```python
from build123d import *

# Parameters (mm, degrees)
CROQUIS1_R              = 9
SALIENTE_EXTRUIR1_DEPTH = 8
CROQUIS3_R              = 11
SALIENTE_EXTRUIR2_DEPTH = 1
SALIENTE_EXTRUIR3_START = 1
CROQUIS4_R              = 11
SALIENTE_EXTRUIR3_DEPTH = 1
CROQUIS5_R              = 4.5
SALIENTE_EXTRUIR4_DEPTH = 6
CROQUIS6_R              = 2.5
CORTAR_EXTRUIR1_DEPTH   = 23.315913604
CROQUIS7_R              = 1
CORTAR_EXTRUIR2_DEPTH   = 18.972200756
CROQUIS8_R              = 1
CORTAR_EXTRUIR5_DEPTH   = 8
MATRIZC1_COUNT          = 20
CHAFL_N1_SIZE           = 0.5


with BuildPart() as part:
    # Croquis1 → Saliente-Extruir1 (new body)
    with BuildSketch(Plane(origin=(0, 0, 0), x_dir=(1, 0, 0), z_dir=(0, 1, 0))):
        with Locations(Location((0, 0, 0), (0, 0, 270))):
            Circle(CROQUIS1_R)
    extrude(amount=SALIENTE_EXTRUIR1_DEPTH)

    # Croquis3 → Saliente-Extruir2 (add)
    with BuildSketch(Plane(origin=(0, 8, 0), x_dir=(1, 0, 0), z_dir=(0, 1, 0))):
        with Locations(Location((0, 0, 0), (0, 0, 270))):
            Circle(CROQUIS3_R)
    extrude(amount=SALIENTE_EXTRUIR2_DEPTH)

    # Croquis4 → Saliente-Extruir3 (add)
    with BuildSketch(Plane.XZ.offset(SALIENTE_EXTRUIR3_START)):
        with Locations(Location((0, 0, 0), (0, 0, 90))):
            Circle(CROQUIS4_R)
    extrude(amount=-SALIENTE_EXTRUIR3_DEPTH)

    # Croquis5 → Saliente-Extruir4 (add)
    with BuildSketch(Plane.XZ.offset(1)):
        with Locations(Location((0, 0, 0), (0, 0, 270))):
            Circle(CROQUIS5_R)
    extrude(amount=SALIENTE_EXTRUIR4_DEPTH)

    # Croquis6 → Cortar-Extruir1 (cut, through all)
    with BuildSketch(Plane(origin=(0, 9, 0), x_dir=(1, 0, 0), z_dir=(0, 1, 0))):
        with Locations(Location((0, 0, 0), (0, 0, 270))):
            Circle(CROQUIS6_R)
    extrude(amount=-CORTAR_EXTRUIR1_DEPTH, mode=Mode.SUBTRACT)

    # Croquis7 → Cortar-Extruir2 (cut, through all)
    with BuildSketch(Plane.XY):
        with Locations((-0.592473365, -4)):
            Circle(CROQUIS7_R)
    extrude(amount=-CORTAR_EXTRUIR2_DEPTH, mode=Mode.SUBTRACT)

    # Croquis8 → Cortar-Extruir5 (cut)
    with BuildSketch(Plane.XZ.offset(-8)):
        with Locations((0, -9)):
            Circle(CROQUIS8_R)
    cortar_extruir5 = extrude(amount=CORTAR_EXTRUIR5_DEPTH, mode=Mode.SUBTRACT)

    # MatrizC1: Cortar-Extruir5 ×20 about axis
    matrizc1_axis = Axis((0, 0, 0), (0, 1, 0))
    for i in range(1, MATRIZC1_COUNT):
        add(cortar_extruir5.rotate(matrizc1_axis, i * 360 / MATRIZC1_COUNT), mode=Mode.SUBTRACT)

    # Chaflán1
    chafl_n1_edges = [part.edges().sort_by_distance(p)[0] for p in [
        (0, -1, 4.5),
        (0, -7, 4.5),
        (0, 9, -2.5),
    ]]
    chamfer(chafl_n1_edges, length=CHAFL_N1_SIZE)


solid = part.part
```
Geometry: final body of the model. Coordinates: model frame, mm. A direction names the side the tool comes from. Coordinates: 2 decimals unless noted, no trailing zeros. Order: outer loops, then holes, each group sorted by start corner. A loop starts at its lowest first (then second) coordinate and runs counter-clockwise, first axis right, second up. Notation, with made-up numbers: (72.25, 35) - (111.25, 35) arc R12 ccw to (111.25, 47) - close; hole circle Ø4 at (82, -30). An arc over 180 degrees is marked (long way). Return JSON: item names as keys, results as strings. Group by question number.
1. Material intervals for line 1 along Y through (x, z) = (0.25, -8.25); line 2 along Z through (x, y) = (-7.75, 5.25); line 3 along X through (y, z) = (-4, -3.4), sorted ascending. Write a range as [from, to].
2. Cut plane A-A (z = 0). Output: boundary loops of the cut face in (x, y).
3. Pin query (flat end, axial travel): pin 1 (5 mm diameter, centred on x = 5, z = -0.5, fed in from -Y); pin 2 (5 mm diameter, centred on x = 5.5, y = -3, fed in from -Z); pin 3 (3 mm diameter, centred on y = 3, z = 5, fed in from -X); pin 4 (3 mm diameter, centred on x = -0.59, y = -4, fed in from +Z). Return the tip coordinate at first contact, or that it passes through.
4. Set-up query: faces 1 (the face through (0, 4, -8)), 2 (the face through (-2.5, 4.1, -7.6)), 3 (the face through (8.89, 3.94, 1.41)), 4 (the face through (1.41, 3.94, -8.89)). Return all of +Z, -Z, +X, -X, +Y, -Y with unobstructed straight access to the full face (end or side cutting, diameter ignored); none if empty.
5. Cut plane C-C (y = -5.75). Output: boundary loops of the cut face in (x, z), plus the area to 3 significant figures.
6. Cut plane B-B (x = 0). Count the separate pieces of the cut face and the enclosed holes in it, plus the area to 3 significant figures.
7. Cut plane D-D (x = 9.5). Output: boundary loops of the cut face in (y, z).
8. Pull-direction query (Z, two-part tool) for faces 5 (the face through (8.89, 3.94, -1.4)), 6 (the face through (7.6, 4.1, -2.5)), 7 (the face through (1.352, -3.965, -4.292)); classes: pulls with the +Z half, pulls with the -Z half, needs draft (parallel to the pull), parting line crosses it, or undercut.
Resolved:
{
 "1": {"line 1": "y = [-1, 0], [8, 9]", "line 2": "z = [-4.41, -3.37], [-2.19, 2.19], [3.37, 4.41]", "line 3": "x = [-2.95, -1.59], [0.41, 2.95]"},
 "2": {"outline": "(-11, -1) - (-5, -1) - (-4.5, -1.5) - (-4.5, -6.5) - (-4, -7) - (-2.5, -7) - (-2.5, 8.5) - (-3, 9) - (-11, 9) - (-11, 8) - (-8, 8) - (-8, 0) - (-11, 0) - close; (2.5, -7) - (4, -7) - (4.5, -6.5) - (4.5, -1.5) - (5, -1) - (11, -1) - (11, 0) - (8, 0) - (8, 8) - (11, 8) - (11, 9) - (3, 9) - (2.5, 8.5) - close"},
 "3": {"pin 1": "stops at y = -7", "pin 2": "stops at z = -10.25", "pin 3": "stops at x = -8.2", "pin 4": "stops at z = 4.5"},
 "4": {"face 1": "-Z", "face 2": "none", "face 3": "+Z, +X", "face 4": "-Z, +X"},
 "5": {"outline": "circle Ø9 at (0, 0); hole circle Ø5 at (0, 0)", "area": "44.0 mm²"},
 "6": {"separate pieces": "3", "enclosed holes": "0", "area": "143 mm²"},
 "7": {"outline": "(-1, -5.55) - (0, -5.55) - (0, 5.55) - (-1, 5.55) - close; (8, -5.55) - (9, -5.55) - (9, 5.55) - (8, 5.55) - close"},
 "8": {"face 5": "pulls with the -Z half", "face 6": "undercut", "face 7": "parting line crosses it"}
}
